```python
from build123d import *

# Parameters (mm, degrees)
TAGLIO_ESTRUSIONE1_REACH             = 10
SCHIZZO2_W                           = 1.5
SCHIZZO2_H                           = 8
TAGLIO_ESTRUSIONE1_DIRECTION_2_REACH = 10
SCHIZZO7_R                           = 3
TAGLIO_ESTRUSIONE2_DEPTH             = 41
FORO_FILETTATO_M8_1_D                = 6.8
FORO_FILETTATO_M8_1_DEPTH            = 12
FORO_FILETTATO_M8_1_TIP              = 2.042926105
SCHIZZO10_OUTSIDE_W                  = 27.192
SCHIZZO10_OUTSIDE_H                  = 27.192
SCHIZZO10_OUTSIDE_R                  = 6.75
TAGLIO_ESTRUSIONE3_DEPTH             = 13


with BuildPart() as part:
    # Schizzo1 → Rivoluzione1 (revolve)
    with BuildSketch(Plane.XY):
        Polygon((0, 0), (-5, 0), (-8, 1.5), (-8, 12), (-6, 12), (-6, 13.5), (-8, 13.5), (-8, 15), (-6, 15), (-6, 16.5), (-8, 16.5), (-8, 18), (-6, 18), (-6, 19.5), (-8, 19.5), (-8, 27), (-8, 40), (0, 40), align=None)
    revolve(axis=Axis((0, 129.407380346, 0), (0, -1, 0)))

    # Schizzo2 → Taglio-Estrusione1 (cut, up to next)
    with BuildSketch(Plane.XY, mode=Mode.PRIVATE) as taglio_estrusione1_sk1:
        with Locations((-7.25, 4)):
            Rectangle(SCHIZZO2_W, SCHIZZO2_H)
    taglio_estrusione1_tool1 = extrude(taglio_estrusione1_sk1.sketch, amount=-TAGLIO_ESTRUSIONE1_REACH, mode=Mode.PRIVATE) & part.part
    add(taglio_estrusione1_tool1.solids().sort_by_distance((-7.25, 4, 0))[0], mode=Mode.SUBTRACT)
    # Schizzo2 → Taglio-Estrusione1 (cut, up to next)
    with BuildSketch(Plane.XY, mode=Mode.PRIVATE) as taglio_estrusione1_sk2:
        with Locations((7.25, 4)):
            Rectangle(SCHIZZO2_W, SCHIZZO2_H)
    taglio_estrusione1_tool2 = extrude(taglio_estrusione1_sk2.sketch, amount=-TAGLIO_ESTRUSIONE1_REACH, mode=Mode.PRIVATE) & part.part
    add(taglio_estrusione1_tool2.solids().sort_by_distance((7.25, 4, 0))[0], mode=Mode.SUBTRACT)

    # Schizzo2 → Taglio-Estrusione1 direction 2 (cut, up to next)
    with BuildSketch(Plane.XY, mode=Mode.PRIVATE) as taglio_estrusione1_direction_2_sk1:
        with Locations((-7.25, 4)):
            Rectangle(SCHIZZO2_W, SCHIZZO2_H)
    taglio_estrusione1_direction_2_tool1 = extrude(taglio_estrusione1_direction_2_sk1.sketch, amount=TAGLIO_ESTRUSIONE1_DIRECTION_2_REACH, mode=Mode.PRIVATE) & part.part
    add(taglio_estrusione1_direction_2_tool1.solids().sort_by_distance((-7.25, 4, 0))[0], mode=Mode.SUBTRACT)
    # Schizzo2 → Taglio-Estrusione1 direction 2 (cut, up to next)
    with BuildSketch(Plane.XY, mode=Mode.PRIVATE) as taglio_estrusione1_direction_2_sk2:
        with Locations((7.25, 4)):
            Rectangle(SCHIZZO2_W, SCHIZZO2_H)
    taglio_estrusione1_direction_2_tool2 = extrude(taglio_estrusione1_direction_2_sk2.sketch, amount=TAGLIO_ESTRUSIONE1_DIRECTION_2_REACH, mode=Mode.PRIVATE) & part.part
    add(taglio_estrusione1_direction_2_tool2.solids().sort_by_distance((7.25, 4, 0))[0], mode=Mode.SUBTRACT)

    # Schizzo7 → Taglio-Estrusione2 (cut, through all)
    with BuildSketch(Plane(origin=(0, 40, 0), x_dir=(1, 0, 0), z_dir=(0, 1, 0))):
        Circle(SCHIZZO7_R)
    extrude(amount=-TAGLIO_ESTRUSIONE2_DEPTH, mode=Mode.SUBTRACT)

    # Foro filettato M8-1
    with Locations(Plane(origin=(0, 0, 0), x_dir=(-1, 0, 0), z_dir=(0, -1, 0))):
        with Locations((0, 0)):
            Hole(FORO_FILETTATO_M8_1_D / 2, depth=FORO_FILETTATO_M8_1_DEPTH)
            with Locations((0, 0, -(FORO_FILETTATO_M8_1_DEPTH + FORO_FILETTATO_M8_1_TIP / 2))):  # 118° drill point
                Cone(0, FORO_FILETTATO_M8_1_D / 2, FORO_FILETTATO_M8_1_TIP, mode=Mode.SUBTRACT)

    # Schizzo10 outside → Taglio-Estrusione3 (cut)
    with BuildSketch(Plane(origin=(0, 40, 0), x_dir=(1, 0, 0), z_dir=(0, 1, 0))):
        Rectangle(SCHIZZO10_OUTSIDE_W, SCHIZZO10_OUTSIDE_H)
        Circle(SCHIZZO10_OUTSIDE_R, mode=Mode.SUBTRACT)
    extrude(amount=-TAGLIO_ESTRUSIONE3_DEPTH, mode=Mode.SUBTRACT)


solid = part.part
```
The listing builds one solid part. Answer for the finished solid, in the listing's coordinates (mm). A direction names the side the tool comes from. Give positions to 0.01 mm unless a question says otherwise; leave off trailing zeros. Loops run counter-clockwise (first coordinate to the right, second up) from the corner with the lowest first, then second, coordinate; pieces in that order, holes last. Notation, with made-up numbers: M -7.75,-32.75 L 12.25,-32.75 A29 ccw 12.25,-8.75 Z; hole C 18,86 d1. An arc over 180 degrees is marked long. One line per item, written item: value.
Q1. A cutting plane is placed at A-A on y = 29.5. Determine the outline of the cut face in (x, z).
Working result:
outline: C 0,0 d13.5; hole C 0,0 d6
Q2. Determine the mould class of faces 1 (the face through (1.73, 23.2, 7.81)), 2 (the face through (6, 13, 0)), 3 (the face through (7, 8, 0)) for opening direction Y: +Y half, -Y half, draft (parallel to the pull), parting line (faces both ways), or undercut.
Working result:
face 1: draft
face 2: undercut
face 3: -Y half
Q3. For faces 4 (the face through (-0.74, 6.08, 3.32)), 5 (the face through (-2, 16.5, -6)), 6 (the face through (-6.5, 4, 0)), 7 (the face through (-4, 27, 6)), determine the directions among +Z, -Z, +X, -X, +Y, -Y from which every point of the face is accessible in a straight line to the end or side of a thin tool.
Working result:
face 4: -Y
face 5: none
face 6: +Z, -Z, -X, -Y
face 7: +Y
Q4. Find the intervals of material crossed by line 1 (Y direction, x = -7, z = -1.25); line 2 (Y direction, x = 1.75, z = -6.25); line 3 (Z direction, x = 0, y = 25.75), in increasing order. Write a range as from..to.
Working result:
line 1: y = 8..12, 13.5..15, 16.5..18, 19.5..27
line 2: y = 0.75..12, 13.5..15, 16.5..18, 19.5..40
line 3: z = -8..-3, 3..8
Q5. Flat-ended cylindrical pins translate along their axes: P1, Ø2, axis at y = 2.5, z = 1, coming from the -X side; P2, Ø2, axis at x = 5.5, z = 5.5, coming from the -Y side; P3, Ø8, axis at x = 0.5, z = 0.5, coming from the +Y side; P4, Ø5.5, axis at x = 0, z = 0, coming from the -Y side. Find the tip coordinate at first contact, or state that the pin passes through.
Working result:
P1: stops at x = -6.5
P2: stops at y = 0.89
P3: stops at y = 40
P4: passes through
